The drawing under review shows one solid part. Ordinate dimensions are in mm from its lowest x, y, z. A direction names the side the tool comes from. Round coordinates to 2 decimals unless told otherwise and drop trailing zeros. Order: outer loops, then holes, each group sorted by start corner. A loop starts at its lowest first (then second) coordinate and runs counter-clockwise, first axis right, second up.
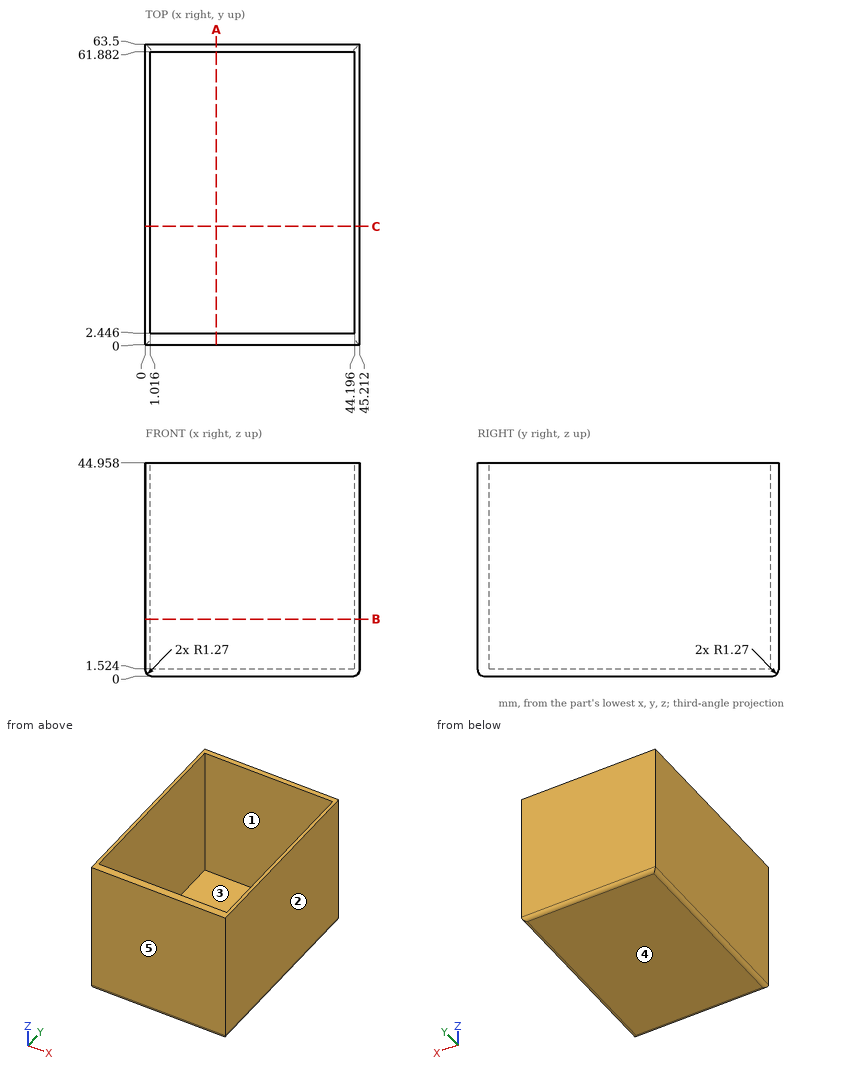
Q1. Mouldability with a two-part tool opening along Y and no side actions: class the marked faces 3, 4 and 5 as +Y half, -Y half, draft (parallel to the pull), parting line (faces both ways), or undercut.
Q2. Wall thickness on line 1 (X direction, y = 28.5, z = 29); line 2 (Y direction, x = 43, z = 3.5); line 3 (Z direction, x = 38, y = 58): over which ranges is each line inside the solid? List them lowest first.
Q3. Take a section at C-C, the plane y = 25. State the section outline as (x, z) points.
Q4. Take a section at B-B, the plane z = 12. State the section outline as (x, y) points.
Q5. Clearance check with a flat-ended pin moving along its axis: pin 1 (8 mm diameter, centred on x = 31, y = 10, fed in from +Z). State where the tip first meets the part, or that it passes through.
Q6. Tool access review of the marked faces 1 and 2: name each direction out of +Z, -Z, +X, -X, +Y, -Y from which nothing blocks a thin tool from reaching the whole face with its end or side.
Q7. Take a section at A-A, the plane x = 15. State the section outline as (y, z) points.
Working result:
1. face 3: undercut
1. face 4: draft
1. face 5: -Y half
2. line 1: x = 0 to 1.02, 44.2 to 45.21
2. line 2: y = 0 to 2.45, 61.88 to 63.5
2. line 3: z = 0 to 1.52
3. outline: (0, 1.27) arc R1.27 ccw to (1.27, 0) - (43.94, 0) arc R1.27 ccw to (45.21, 1.27) - (45.21, 44.96) - (44.2, 44.96) - (44.2, 1.52) - (1.02, 1.52) - (1.02, 44.96) - (0, 44.96) - close
4. outline: (0, 0) - (45.21, 0) - (45.21, 63.5) - (0, 63.5) - close; hole (1.02, 2.45) - (44.2, 2.45) - (44.2, 61.88) - (1.02, 61.88) - close
5. pin 1: stops at z = 1.52
6. face 1: +Z
6. face 2: +Z, -Z, +X, +Y, -Y
7. outline: (0, 1.27) arc R1.27 ccw to (1.27, 0) - (62.23, 0) arc R1.27 ccw to (63.5, 1.27) - (63.5, 44.96) - (61.88, 44.96) - (61.88, 1.52) - (2.45, 1.52) - (2.45, 44.96) - (0, 44.96) - close
